from build123d import *

# Parameters (mm, degrees)
F1_DEPTH  = 50
F3_DEPTH  = 1
F5_DEPTH  = 1
F6_DEPTH  = 1
F7_SIZE   = 0.99999
F9_DEPTH  = 37.5
F10_DEPTH = 12.5
F11_R     = 20


# Not quite as in the source:
# - a fillet or chamfer is up to 0.001 mm smaller than in the source, because OpenCascade refuses the exact size


with BuildPart() as f1:
    # F0 (on Top) → F1 (new body)
    with BuildSketch(Plane.XY):
        with BuildLine():
            Line((-59, 0), (0, 0))
            Line((0, 0), (59, 0))
            ThreePointArc((59, 0), (60.4142135624, -0.5857864376), (61, -2))
            Line((61, -2), (61, -22.5753318518))
            Line((61, -22.5753318518), (62, -22.5753318518))
            Line((62, -22.5753318518), (62, 1))
            Line((62, 1), (0, 1))
            Line((0, 1), (-62, 1))
            Line((-62, 1), (-62, -22.5753318518))
            Line((-62, -22.5753318518), (-61, -22.5753318518))
            Line((-61, -22.5753318518), (-61, -2))
            ThreePointArc((-61, -2), (-60.4142135624, -0.5857864376), (-59, 0))
        make_face()
    extrude(amount=F1_DEPTH)

    # F2 (on face) → F3 (join)
    with BuildSketch(Plane(origin=(-62, 0, 0), x_dir=(0, -1, 0), z_dir=(-1, 0, 0))):
        Polygon((74.8511105776, 0), (22.5753318518, 50), (22.5753318518, 0), align=None)
    extrude(amount=-F3_DEPTH)

    # F4 (on face) → F5 (join)
    with BuildSketch(Plane.YZ.offset(62)):
        Polygon((-22.5753318518, 0), (-22.5753318518, 50), (-74.9809518456, 0), align=None)
    extrude(amount=-F5_DEPTH)

    # F0 (on Top) → F6 (join)
    with BuildSketch(Plane.XY):
        Polygon((62, 1), (62, -22.5753318518), (62, -75), (63, -75), (63, 1), align=None)
        Polygon((-62, -75), (-62, -22.5753318518), (-62, 1), (-63, 1), (-63, -75), align=None)
    extrude(amount=F6_DEPTH)

    # F7 (size 1 in the source; OpenCascade refuses exactly that, so slightly less here)
    f7_edges = [f1.edges().sort_by_distance(p)[0] for p in [
        (62.5, -75, 1),
        (-62.5, -75, 1),
    ]]
    chamfer(f7_edges, length=F7_SIZE)

    # F8 (on Right) → F9 (join, symmetric)
    with BuildSketch(Plane.YZ):
        with BuildLine():
            Line((1, -12.3380962103), (1, 0))
            Line((1, 0), (-6.78e-08, 0))
            Line((-6.78e-08, 0), (-6.78e-08, -12.3380962103))
            ThreePointArc((-6.78e-08, -12.3380962103), (-4.5657106986, -20.1698953121), (-13.6304617639, -20.0555324836))
            Line((-13.6304617639, -20.0555324836), (-37.0563493496, -5.9999999322))
            Line((-37.0563493496, -5.9999999322), (-44.3333333333, -5.9999999322))
            ThreePointArc((-44.3333333333, -5.9999999322), (-45.8844675886, -6.5087526502), (-46.8329720249, -7.8373557287))
            Line((-46.8329720249, -7.8373557287), (-45.8785471313, -8.1358071621))
            ThreePointArc((-45.8785471313, -8.1358071621), (-45.2922055343, -7.3144981402), (-44.3333333333, -7))
            Line((-44.3333333333, -7), (-37.3333333333, -7))
            Line((-37.3333333333, -7), (-14.1449575543, -20.9130254674))
            ThreePointArc((-14.1449575543, -20.9130254674), (-4.0730118502, -21.0400952778), (1, -12.3380962103))
        make_face()
    extrude(amount=F9_DEPTH, both=True)

    # F8 (on Right) → F10 (cut, symmetric)
    with BuildSketch(Plane.YZ):
        with BuildLine():
            Line((1, -12.3380962103), (1, 0))
            Line((1, 0), (-6.78e-08, 0))
            Line((-6.78e-08, 0), (-6.78e-08, -12.3380962103))
            ThreePointArc((-6.78e-08, -12.3380962103), (-4.5657106986, -20.1698953121), (-13.6304617639, -20.0555324836))
            Line((-13.6304617639, -20.0555324836), (-37.0563493496, -5.9999999322))
            Line((-37.0563493496, -5.9999999322), (-44.3333333333, -5.9999999322))
            ThreePointArc((-44.3333333333, -5.9999999322), (-45.8844675886, -6.5087526502), (-46.8329720249, -7.8373557287))
            Line((-46.8329720249, -7.8373557287), (-45.8785471313, -8.1358071621))
            ThreePointArc((-45.8785471313, -8.1358071621), (-45.2922055343, -7.3144981402), (-44.3333333333, -7))
            Line((-44.3333333333, -7), (-37.3333333333, -7))
            Line((-37.3333333333, -7), (-14.1449575543, -20.9130254674))
            ThreePointArc((-14.1449575543, -20.9130254674), (-4.0730118502, -21.0400952778), (1, -12.3380962103))
        make_face()
    extrude(amount=F10_DEPTH, both=True, mode=Mode.SUBTRACT)

    # F11
    f11_edges = [f1.edges().sort_by_distance(p)[0] for p in [
        (-61.5, -22.575332, 50),
        (61.5, -22.575332, 50),
    ]]
    fillet(f11_edges, radius=F11_R)


solid = f1.part
Input: part model. Units: mm. Frame: model coordinates. A direction names the side the tool comes from. Give positions to 0.01 mm unless a question says otherwise; leave off trailing zeros. Write each loop counter-clockwise with the first axis right and the second up, starting at its lowest first coordinate (ties: lowest second). Pieces come first, ordered by that corner, then holes. Notation, with made-up numbers: (79.5, 55.5) -> (138.5, 55.5) arc R34 cw to (138.5, 93.5) -> close; hole circle Ø9 at (64, -14.5). An arc over 180 degrees is marked (long way). Use one line per item in the form item = value. Start each with the question number.
1) Section query D-D on z = 33. Return the cut outline in (x, y).
2) Section query C-C on y = -55.5. Return the cut outline in (x, z).
3) Section query B-B on x = -22.5. Return the cut outline in (y, z), then the cut area to 3 significant figures.
4) Pin query (flat end, axial travel): pin 1 (3.5 mm diameter, centred on x = -19.5, y = -42, fed in from -Z); pin 2 (15 mm diameter, centred on y = -47, z = 35.5, fed in from -X); pin 3 (0.8 mm diameter, centred on x = -62.5, y = -42, fed in from +Z); pin 4 (4 mm diameter, centred on x = -32.5, y = -50, fed in from -Z). Return the tip coordinate at first contact, or that it passes through.
5) Section query A-A on y = -34. Return the cut outline in (x, z), then the cut area to 3 significant figures.
6) Draft query along Y for faces 6 (the cylindrical face through (-25, -4, -21)), 7 (the cylindrical face through (25.175, -4.45, -20.104)), 8 (the flat face through (25, -41, -7)), 9 (the flat face through (-25, -41, -6)). Return one class per face: pulls with the +Y half, pulls with the -Y half, needs draft (parallel to the pull), parting line crosses it, or undercut.
7) Set-up query: faces 1 (the flat face through (-12.5, -19.5, -16.9)), 2 (the flat face through (37.5, -19.5, -16.9)), 3 (the flat face through (25.175, -25.179, -13.126)), 4 (the flat face through (-37.5, -19.5, -16.9)), 5 (the cylindrical face through (-24.82, -45.87, -6.5)). Return all of +Z, -Z, +X, -X, +Y, -Y with unobstructed straight access to the full face (end or side cutting, diameter ignored); none if empty.
8) Ray query, probe 1 along X at (y, z) = (-30.5, 19); probe 2 along Y at (x, z) = (25.5, 30.5); probe 3 along Z at (x, y) = (-25, -38). Return the intervals inside material, ascending. Write a range as from..to.
Outcome:
q1.outline = (-62, -40.35) -> (-61, -40.35) -> (-61, -2) arc R2 cw to (-59, 0) -> (59, 0) arc R2 cw to (61, -2) -> (61, -40.39) -> (62, -40.39) -> (62, 1) -> (-62, 1) -> close
q2.outline = (-63, 0) -> (-61, 0) -> (-61, 18.51) -> (-62, 18.51) -> (-62, 1) -> (-63, 1) -> close; (61, 0) -> (63, 0) -> (63, 1) -> (62, 1) -> (62, 18.59) -> (61, 18.59) -> close
q3.outline = (-46.83, -7.84) -> (-45.88, -8.14) arc R1.62 cw to (-44.33, -7) -> (-37.33, -7) -> (-14.14, -20.91) arc R10 ccw to (1, -12.34) -> (1, 50) -> (0, 50) -> (0, -12.34) arc R9 cw to (-13.63, -20.06) -> (-37.06, -6) -> (-44.33, -6) arc R2.62 ccw to start
q3.area = 119 mm^2
q4.pin_1 = -7
q4.pin_2 = -62
q4.pin_3 = 1
q4.pin_4 = through
q5.outline = (-63, 0) -> (-61, 0) -> (-61, 39.07) -> (-62, 39.07) -> (-62, 1) -> (-63, 1) -> close; (-37.5, -9) -> (-12.5, -9) -> (-12.5, -7.83) -> (-37.5, -7.83) -> close; (12.5, -9) -> (37.5, -9) -> (37.5, -7.83) -> (12.5, -7.83) -> close; (61, 0) -> (63, 0) -> (63, 1) -> (62, 1) -> (62, 39.1) -> (61, 39.1) -> close
q5.area = 138 mm^2
q6.face_6 = parting line crosses it
q6.face_7 = undercut
q6.face_8 = undercut
q6.face_9 = needs draft
q7.face_1 = -Z, +Y, -Y
q7.face_2 = -Z, +X, +Y, -Y
q7.face_3 = +Z, +X, -X
q7.face_4 = -Z, -X, +Y, -Y
q7.face_5 = +Z, +X, -X, -Y
q8.probe_1 = -62..-61, 61..62
q8.probe_2 = 0..1
q8.probe_3 = -7..-6
